```python
from build123d import *

# Parameters (mm, degrees)
F1_DEPTH  = 3.8
F2_R      = 1.5
F3_W      = 68
F3_H      = 33
F4_DEPTH  = 21.7
F5_W      = 63.5
F5_H      = 28.6
F6_DEPTH  = 21.7
F7_R      = 3
F9_DEPTH  = 2
F10_R     = 1
F8_W      = 57.9
F8_H      = 12.6
F11_DEPTH = 0.75


with BuildPart() as f1:
    # F0 (on Top) → F1 (new body)
    with BuildSketch(Plane.XY):
        with BuildLine():
            Line((-34.45, -19.55), (34.45, -19.55))
            ThreePointArc((34.45, -19.55), (36.57132, -18.67132), (37.45, -16.55))
            Line((37.45, -16.55), (37.45, 16.55))
            ThreePointArc((37.45, 16.55), (36.57132, 18.67132), (34.45, 19.55))
            Line((34.45, 19.55), (-34.45, 19.55))
            ThreePointArc((-34.45, 19.55), (-36.57132, 18.67132), (-37.45, 16.55))
            Line((-37.45, 16.55), (-37.45, -16.55))
            ThreePointArc((-37.45, -16.55), (-36.57132, -18.67132), (-34.45, -19.55))
        make_face()
    extrude(amount=F1_DEPTH)

    # F2
    f2_edges = [f1.edges().sort_by_distance(p)[0] for p in [
        (0, -19.55, 3.8),
        (36.57132, -18.67132, 3.8),
        (37.45, 0, 3.8),
        (36.57132, 18.67132, 3.8),
        (0, 19.55, 3.8),
        (-36.57132, 18.67132, 3.8),
        (-37.45, 0, 3.8),
        (-36.57132, -18.67132, 3.8),
    ]]
    fillet(f2_edges, radius=F2_R)

    # F3 (on face) → F4 (join)
    with BuildSketch(Plane(origin=(0, 0, 0), x_dir=(1, 0, 0), z_dir=(0, 0, -1))):
        Rectangle(F3_W, F3_H)
    extrude(amount=F4_DEPTH)

    # F5 (on face) → F6 (join)
    with BuildSketch(Plane(origin=(0, 0, -21.7), x_dir=(1, 0, 0), z_dir=(0, 0, -1))):
        Rectangle(F5_W, F5_H)
    extrude(amount=F6_DEPTH)

    # F7
    f7_edges = [f1.edges().sort_by_distance(p)[0] for p in [
        (0, -14.3, -43.4),
        (0, 14.3, -43.4),
    ]]
    fillet(f7_edges, radius=F7_R)

    # F8 (on face) → F9 (join)
    with BuildSketch(Plane.XY.offset(3.8)):
        with BuildLine():
            Line((21.95, 7.55), (27.45, 7.55))
            ThreePointArc((27.45, 7.55), (28.51066, 7.98934), (28.95, 9.05))
            Line((28.95, 9.05), (28.95, 10.05))
            ThreePointArc((28.95, 10.05), (28.51066, 11.11066), (27.45, 11.55))
            Line((27.45, 11.55), (21.95, 11.55))
            ThreePointArc((21.95, 11.55), (20.88934, 11.11066), (20.45, 10.05))
            Line((20.45, 10.05), (20.45, 9.05))
            ThreePointArc((20.45, 9.05), (20.88934, 7.98934), (21.95, 7.55))
        make_face()
        with BuildLine():
            ThreePointArc((-21.95, 7.55), (-20.88934, 7.98934), (-20.45, 9.05))
            Line((-20.45, 9.05), (-20.45, 10.05))
            ThreePointArc((-20.45, 10.05), (-20.88934, 11.11066), (-21.95, 11.55))
            Line((-21.95, 11.55), (-27.45, 11.55))
            ThreePointArc((-27.45, 11.55), (-28.51066, 11.11066), (-28.95, 10.05))
            Line((-28.95, 10.05), (-28.95, 9.05))
            ThreePointArc((-28.95, 9.05), (-28.51066, 7.98934), (-27.45, 7.55))
            Line((-27.45, 7.55), (-21.95, 7.55))
        make_face()
    extrude(amount=F9_DEPTH)

    # F10
    f10_edges = [f1.edges().sort_by_distance(p)[0] for p in [
        (20.88934, 7.98934, 5.8),
        (24.7, 7.55, 5.8),
        (28.51066, 7.98934, 5.8),
        (28.95, 9.55, 5.8),
        (28.51066, 11.11066, 5.8),
        (24.7, 11.55, 5.8),
        (20.88934, 11.11066, 5.8),
        (20.45, 9.55, 5.8),
        (-20.88934, 7.98934, 5.8),
        (-20.45, 9.55, 5.8),
        (-20.88934, 11.11066, 5.8),
        (-24.7, 11.55, 5.8),
        (-28.51066, 11.11066, 5.8),
        (-28.95, 9.55, 5.8),
        (-28.51066, 7.98934, 5.8),
        (-24.7, 7.55, 5.8),
    ]]
    fillet(f10_edges, radius=F10_R)

    # F8 (on face) → F11 (cut)
    with BuildSketch(Plane.XY.offset(3.8)):
        with Locations((0, -4.75)):
            Rectangle(F8_W, F8_H)
    extrude(amount=-F11_DEPTH, mode=Mode.SUBTRACT)


solid = f1.part
```
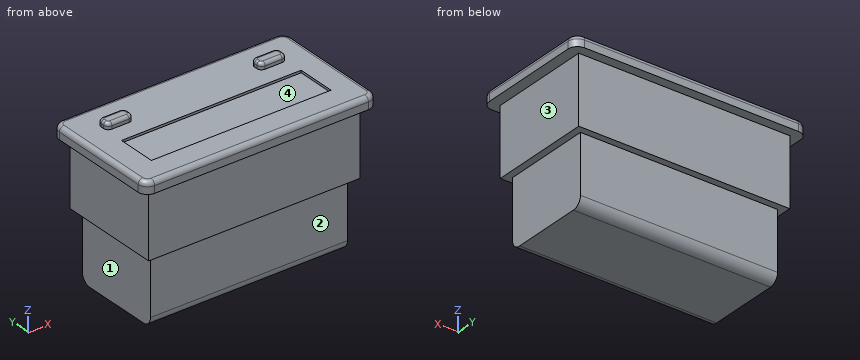
Check sheet for the modelled part. Datum: model origin and axes. Units: mm. Face numbers are marked on the shaded views. A direction names the side the tool comes from. Coordinates: 2 decimals unless noted, no trailing zeros. Order: outer loops, then holes, each group sorted by start corner. A loop starts at its lowest first (then second) coordinate and runs counter-clockwise, first axis right, second up. Notation, with made-up numbers: M 19,58.25 L 75,58.25 A22 cw 75,83.25 Z; hole C 68.25,71.25 d10. An arc over 180 degrees is marked long. Write each question's results on one line, items separated by ' | '. Start each with the question number.
1. Go/stop test with flat-tipped pins: P1, Ø0.8, axis at x = -23.5, z = 4.5, coming from the +Y side; P2, Ø8, axis at y = -13.5, z = -25, coming from the +X side; P3, Ø5, axis at y = -10.5, z = -15, coming from the -X side. Record where each tip stops, or that it passes through.
2. Cross-section at A-A on x = -25.5. Record the cut outline in (y, z).
3. Cross-section at B-B on y = -10. Record the cut outline in (x, z), and give its area (3 significant figures).
4. Cross-section at D-D on x = -18. Record the cut outline in (y, z), and give its area (3 significant figures).
5. Material ranges on probe 1 along Y at (x, z) = (9, -12); probe 2 along Y at (x, z) = (14, -33.5); probe 3 along X at (y, z) = (-10.5, -13), recorded low to high.
6. Access from +Z, -Z, +X, -X, +Y, -Y to the whole of each face (thin tool, end or side, straight path). Record for the marked faces 1, 2, 3 and 4.
7. Cross-section at C-C on z = -38.5. Record the cut outline in (x, y), and give its area (3 significant figures).
Checks:
1) P1: stops at y = 11.55 | P2: stops at x = 34 | P3: stops at x = -34
2) outline: M -19.55,0 L -16.5,0 L -16.5,-21.7 L -14.3,-21.7 L -14.3,-40.4 A3 ccw -11.3,-43.4 L 11.3,-43.4 A3 ccw 14.3,-40.4 L 14.3,-21.7 L 16.5,-21.7 L 16.5,0 L 19.55,0 L 19.55,2.3 A1.5 ccw 18.05,3.8 L 11.55,3.8 L 11.55,4.8 A1 ccw 10.55,5.8 L 8.55,5.8 A1 ccw 7.55,4.8 L 7.55,3.8 L 1.55,3.8 L 1.55,3.05 L -11.05,3.05 L -11.05,3.8 L -18.05,3.8 A1.5 ccw -19.55,2.3 Z
3) outline: M -37.45,0 L -34,0 L -34,-21.7 L -31.75,-21.7 L -31.75,-43.4 L 31.75,-43.4 L 31.75,-21.7 L 34,-21.7 L 34,0 L 37.45,0 L 37.45,2.3 A1.5 ccw 35.95,3.8 L 28.95,3.8 L 28.95,3.05 L -28.95,3.05 L -28.95,3.8 L -35.95,3.8 A1.5 ccw -37.45,2.3 Z | area: 3,090 mm²
4) outline: M -19.55,0 L -16.5,0 L -16.5,-21.7 L -14.3,-21.7 L -14.3,-40.4 A3 ccw -11.3,-43.4 L 11.3,-43.4 A3 ccw 14.3,-40.4 L 14.3,-21.7 L 16.5,-21.7 L 16.5,0 L 19.55,0 L 19.55,2.3 A1.5 ccw 18.05,3.8 L 1.55,3.8 L 1.55,3.05 L -11.05,3.05 L -11.05,3.8 L -18.05,3.8 A1.5 ccw -19.55,2.3 Z | area: 1,470 mm²
5) probe 1: y = -16.5 to 16.5 | probe 2: y = -14.3 to 14.3 | probe 3: x = -34 to 34
6) face 1: -Z, -X, +Y, -Y | face 2: -Z, +X, -X, -Y | face 3: -Z, +X, +Y, -Y | face 4: +Z
7) outline: M -31.75,-14.3 L 31.75,-14.3 L 31.75,14.3 L -31.75,14.3 Z | area: 1,820 mm²
